```python
from build123d import *

# Parameters (mm, degrees)
SKETCH_1_W     = 12
SKETCH_1_H     = 2.5
CHAMFER_1_SIZE = 0.1


with BuildPart() as part:
    # 草图1 → 旋转1 (revolve)
    with BuildSketch(Plane.XY, mode=Mode.PRIVATE) as revolve_1_sk:
        with Locations((0, 1.25)):
            Rectangle(SKETCH_1_W, SKETCH_1_H)
    revolve(revolve_1_sk.sketch.rotate(Axis((-6, 0, 0), (1, 0, 0)), 180), axis=Axis((-6, 0, 0), (1, 0, 0)))

    # 草图3 → Hole Wizard 378 (revolve, cut)
    with BuildSketch(Plane(origin=(-6, 0, 0), x_dir=(0, 0, 1), z_dir=(0, 1, 0))):
        Polygon((0, 0), (0, 10.751075774), (1.25, 10), (1.25, 0), align=None)
    hole_wizard_378 = revolve(axis=Axis((-12.35, 0, 0), (1, 0, 0)), mode=Mode.SUBTRACT)

    # 镜向1: Hole Wizard 378 across plane
    add(hole_wizard_378.mirror(Plane(origin=(0, 0, 0), x_dir=(0, 0, 1), z_dir=(1, 0, 0))), mode=Mode.SUBTRACT)

    # 倒角1
    chamfer_1_edges = [part.edges().sort_by_distance(p)[0] for p in [
        (-6, 2.5, 0),
        (6, 2.5, 0),
    ]]
    chamfer(chamfer_1_edges, length=CHAMFER_1_SIZE)


solid = part.part
```
Model file for the job. Use its own axes, mm. Round coordinates to 2 decimals unless told otherwise and drop trailing zeros. Write each loop counter-clockwise with the first axis right and the second up, starting at its lowest first coordinate (ties: lowest second). Pieces come first, ordered by that corner, then holes. Notation, with made-up numbers: M 65,57 L 118,57 A19 ccw 118,81 Z; hole C 65,45.5 d4. An arc over 180 degrees is marked long. Put each result on its own line as item: value.
Item 1: Cut at C-C (x = 5.25). List the corners of the cut face in (y, z), and give its area (3 significant figures).
Responses:
outline: C 0,0 d5; hole C 0,0 d2.5
area: 14.7 mm²
Item 2: Flat gauge pin, fed straight in: P1, Ø1, axis at x = 1.5, y = -1, coming from the -Z side. Where does the tip first touch, or does it go through?
Responses:
P1: z = -2.45
Item 3: Cut at A-A (y = 0). List the corners of the cut face in (x, z), and give its area (3 significant figures).
Responses:
outline: M -6,-2.4 L -5.9,-2.5 L 5.9,-2.5 L 6,-2.4 L 6,-1.25 L -6,-1.25 Z; M -6,1.25 L 6,1.25 L 6,2.4 L 5.9,2.5 L -5.9,2.5 L -6,2.4 Z
area: 30.0 mm²
Item 4: Probe L1, parallel to Z at x = -4.8, y = 0; L2, parallel to Y at x = -1.5, z = -0.75; L3, parallel to Y at x = -2.75, z = -0.85. List the from-to ranges inside material, lowest first. Write a range as from..to.
Responses:
L1: -2.5..-1.25, 1.25..2.5
L2: -2.38..-1, 1..2.38
L3: -2.35..-0.92, 0.92..2.35
